from build123d import *

# Parameters (mm, degrees)
SKETCH1_W           = 5
SKETCH1_H           = 6.6
BOSS_EXTRUDE1_REACH = 64.005
SKETCH21_R          = 5
BOSS_EXTRUDE2_REACH = 78.152
SKETCH22_R          = 5
CUT_EXTRUDE3_DEPTH  = 6.6
CUT_EXTRUDE4_DEPTH  = 6.6
CUT_EXTRUDE5_DEPTH  = 6.6
CHAMFER2_SIZE       = 0.5


with BuildPart() as part:
    # Sketch1 → Revolve-Thin1 (revolve)
    with BuildSketch(Plane(origin=(0, 0, 0), x_dir=(1, 0, 0), z_dir=(0, 1, 0))):
        with Locations((-2.5, 20.8)):
            Rectangle(SKETCH1_W, SKETCH1_H)
    revolve(axis=Axis((0, 0, -17.5), (0, 0, -1)))

    # Sketch21 → Boss-Extrude1 (add, up to next)
    with BuildSketch(Plane(origin=(-35.950232756, 0, -65.780747057), x_dir=(0.877503712, 0, -0.479569845), z_dir=(0.479569845, 0, 0.877503712)), mode=Mode.PRIVATE) as boss_extrude1_sk1:
        with Locations((9.975052777, 0)):
            Circle(SKETCH21_R)
    boss_extrude1_tool1 = extrude(boss_extrude1_sk1.sketch, amount=BOSS_EXTRUDE1_REACH, mode=Mode.PRIVATE) - part.part
    add(boss_extrude1_tool1.solids().sort_by_distance((-27.197087, 0, -70.564482))[0])

    # Sketch22 → Boss-Extrude2 (add, up to next)
    with BuildSketch(Plane(origin=(36.517428466, 0, -67.14845845), x_dir=(0.878494382, 0, 0.477752677), z_dir=(-0.477752677, 0, 0.878494382)), mode=Mode.PRIVATE) as boss_extrude2_sk1:
        with Locations((-9.937255677, 0)):
            Circle(SKETCH22_R)
    boss_extrude2_tool1 = extrude(boss_extrude2_sk1.sketch, amount=BOSS_EXTRUDE2_REACH, mode=Mode.PRIVATE) - part.part
    add(boss_extrude2_tool1.solids().sort_by_distance((27.787605, 0, -71.896009))[0])

    # Sketch29 → Cut-Extrude3 (cut)
    with BuildSketch(Plane(origin=(-35.950232756, 0, -65.780747057), x_dir=(-0.877503712, 0, 0.479569845), z_dir=(-0.479569845, 0, -0.877503712))):
        Polygon((-7.089955208, 1.433531311), (-9.773978525, 3.215333442), (-12.659076094, 1.781802131), (-12.860150346, -1.433531311), (-10.176127029, -3.215333442), (-7.29102946, -1.781802131), align=None)
    extrude(amount=-CUT_EXTRUDE3_DEPTH, mode=Mode.SUBTRACT)

    # Sketch30 → Cut-Extrude4 (cut)
    with BuildSketch(Plane(origin=(36.517428466, 0, -67.14845845), x_dir=(-0.878494382, 0, -0.477752677), z_dir=(0.477752677, 0, -0.878494382))):
        Polygon((12.621278993, 1.781802131), (9.736181425, 3.215333442), (7.052158108, 1.433531311), (7.25323236, -1.781802131), (10.138329929, -3.215333442), (12.822353245, -1.433531311), align=None)
    extrude(amount=-CUT_EXTRUDE4_DEPTH, mode=Mode.SUBTRACT)

    # Sketch18 → Cut-Extrude5 (cut)
    with BuildSketch(Plane.XY.offset(-17.5)):
        Polygon((1.610807251, 2.79), (-1.610807251, 2.79), (-3.221614502, 0), (-1.610807251, -2.79), (1.610807251, -2.79), (3.221614502, 0), align=None)
    extrude(amount=-CUT_EXTRUDE5_DEPTH, mode=Mode.SUBTRACT)

    # Chamfer2
    chamfer2_edges = [part.edges().sort_by_distance(p)[0] for p in [
        (-29.640549045, -0.17413541, -69.229090352),
        (-28.551150535, 2.324432377, -69.824464101),
        (-26.107688412, 2.498567787, -71.159855321),
        (-24.753624798, 0.17413541, -71.899872792),
        (-25.843023308, -2.324432377, -71.304499043),
        (-28.286485432, -2.498567787, -69.969107823),
        (25.341384472, 0.17413541, -73.226340155),
        (26.696976775, 2.498567787, -72.489126731),
        (29.143197481, 2.324432377, -71.158795526),
        (30.233825884, -0.17413541, -70.565677745),
        (28.87823358, -2.498567787, -71.302891169),
        (26.432012874, -2.324432377, -72.633222374),
        (2.416210877, 1.395, -17.5),
        (0, 2.79, -17.5),
        (-2.416210877, 1.395, -17.5),
        (-2.416210877, -1.395, -17.5),
        (0, -2.79, -17.5),
        (2.416210877, -1.395, -17.5),
    ]]
    chamfer(chamfer2_edges, length=CHAMFER2_SIZE)


solid = part.part
Build history of the part. All positions in model axes, mm. A direction names the side the tool comes from. Coordinates: 2 decimals unless noted, no trailing zeros. Write item = value, one per line. Start each with the question number.
1) 3-axis set-ups, long thin cutter, end or side, ignore diameter. For faces 4 (the face through (0, 0, -24.1)), 5 (the face through (-25.91, 2.73, -70.98)), 6 (the face through (-24.14, -2.31, -68.24)): which of +Z, -Z, +X, -X, +Y, -Y reach the whole face in a straight line?
2) Wall check: line 1 along X through (y, z) = (-3, -67.5); line 2 along X through (y, z) = (2.75, -65); line 3 along X through (y, z) = (-1.5, -32). Give the ranges that are in metal, low to high. Write a range as from..to.
3) Two-plate mould, pull along Y, no slides. Class faces 1 (the face through (-2.62, 1.54, -17.75)), 2 (the face through (0, 5, -23)), 3 (the face through (-18.172, 0.22, -43.635)): pulls with the +Y half, pulls with the -Y half, needs draft (parallel to the pull), parting line crosses it, or undercut.
4) Flat gauge pins, fed straight in: pin 1 Ø4 at (x, y) = (-3.5, 2) entering from -Z; pin 2 Ø3 at (x, y) = (-1, 0.5) entering from +Z; pin 3 Ø5 at (x, z) = (-23, -56.5) entering from +Y. Where does each tip first touch, or does it go through?
From the geometry:
q1.face_4 = +Z
q1.face_5 = -Z, -X
q1.face_6 = none
q2.line_1 = -30.08..-25.79, -24.92..-20.96, 20.84..24.8, 25.66..29.95
q2.line_2 = -28.91..-25.18, -23.62..-19.4, 19.28..28.79
q2.line_3 = -11.56..-0.69, 0.66..11.52
q3.face_1 = undercut
q3.face_2 = pulls with the +Y half
q3.face_3 = parting line crosses it
q4.pin_1 = -40.7
q4.pin_2 = -24.1
q4.pin_3 = 4.97
